```python
from build123d import *

# Parameters (mm, degrees)
BOSS_EXTRUDE1_DEPTH = 6
SKETCH4_R           = 6
BOSS_EXTRUDE2_DEPTH = 6
SKETCH3_R           = 2
SKETCH3_R_2         = 6
CUT_EXTRUDE1_DEPTH  = 279.190582155


with BuildPart() as part:
    # Sketch2 → Boss-Extrude1 (new body)
    with BuildSketch(Plane(origin=(0, 0, 0), x_dir=(0, 0, -1), z_dir=(1, 0, 0))):
        Polygon((0, 277), (6, 277), (6, 0), (0, 0), (-25, 25), (-25, 252), align=None)
    extrude(amount=BOSS_EXTRUDE1_DEPTH)

    # Sketch4 → Boss-Extrude2 (add)
    with BuildSketch(Plane(origin=(6, 0, 0), x_dir=(0, 0, -1), z_dir=(1, 0, 0))):
        with Locations((-12, 265)):
            Circle(SKETCH4_R)
    extrude(amount=-BOSS_EXTRUDE2_DEPTH)

    # Sketch3 → Cut-Extrude1 (cut, through all)
    with BuildSketch(Plane(origin=(6, 0, 0), x_dir=(0, 0, -1), z_dir=(1, 0, 0))):
        with Locations((-12, 265)):
            Circle(SKETCH3_R)
        with Locations((-12, 12)):
            Circle(SKETCH3_R_2)
    extrude(amount=-CUT_EXTRUDE1_DEPTH, mode=Mode.SUBTRACT)


solid = part.part
```
Work out the finished part from the listing and answer in its coordinate system (mm). A direction names the side the tool comes from. Give positions to 0.01 mm unless a question says otherwise; leave off trailing zeros. Loops run counter-clockwise (first coordinate to the right, second up) from the corner with the lowest first, then second, coordinate; pieces in that order, holes last. Notation, with made-up numbers: (44, 73) -> (52, 73) arc R5 ccw to (52, 80) -> close; hole circle Ø2 at (56, 33.25). An arc over 180 degrees is marked (long way). Put each result on its own line as item: value. Start each with the question number.
Item 1: The mould has two halves that part along Z. Classify faces 4 (the face through (3.042, 16.148, 7.665)), 5 (the face through (3, 137, 25)), 6 (the face through (3, 277, -3)): released by +Z, released by -Z, zero draft, split by the parting line, or undercut.
Item 2: The part is cut by section B-B (y = 12). Give the vertices of the cut face in (x, z), then the cut area to 3 significant figures.
Item 3: The part is cut by section A-A (x = 4.55). Give the vertices of the cut face in (y, z), then the cut area to 3 significant figures.
Item 4: The part is cut by section C-C (z = 21.5). Give the vertices of the cut face in (x, y).
Item 5: Which of the six approach directions +Z, -Z, +X, -X, +Y, -Y give full straight-line access (tool end or side, diameter ignored) to faces 1 (the face through (3, 273, 4)), 2 (the face through (3, 256, 21)), 3 (the face through (3, 0, -3))?
Item 6: Find the intervals of material crossed by L1, parallel to Z at x = 4.45, y = 265; L2, parallel to Y at x = 1.55, z = 12; L3, parallel to Y at x = 4.5, z = 11.5, in increasing order. Write a range as [from, to].
Item 7: This flat-tipped pin is pushed along its axis until it touches: P1, Ø1, axis at x = 1.5, z = 7, coming from the -Y side. Where does it stop, or does it pass through?
Answers below:
1. face 4: undercut
1. face 5: released by +Z
1. face 6: zero draft
2. outline: (0, -6) -> (6, -6) -> (6, 6) -> (0, 6) -> close
2. area: 72.0 mm2
3. outline: (0, -6) -> (277, -6) -> (277, 0) -> (269.24, 7.76) arc R6 ccw to (260.76, 16.24) -> (252, 25) -> (25, 25) -> (16.24, 16.24) arc R6 cw to (7.76, 7.76) -> (0, 0) -> close; hole circle Ø4 at (265, 12)
3. area: 7,950 mm2
4. outline: (0, 21.5) -> (6, 21.5) -> (6, 255.5) -> (0, 255.5) -> close
5. face 1: +X, -X, +Y
5. face 2: +Z, +X, -X
5. face 3: +Z, -Z, +X, -X, -Y
6. L1: [-6, 10], [14, 18]
6. L2: [18, 263], [267, 271]
6. L3: [17.98, 263.06], [266.94, 270.98]
7. P1: y = 6.5
